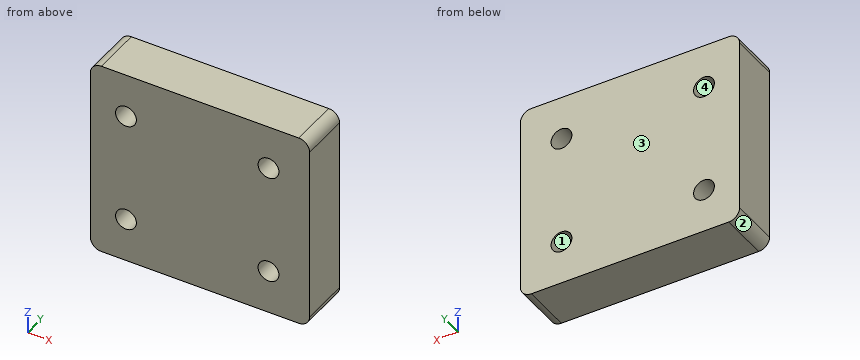
```python
from build123d import *

# Parameters (mm, degrees)
SKETCH1_W           = 40
SKETCH1_H           = 36
BOSS_EXTRUDE1_DEPTH = 9
SKETCH2_R           = 1.9
CUT_EXTRUDE1_DEPTH  = 10
FILLET1_R           = 2


with BuildPart() as part:
    # Sketch1 → Boss-Extrude1 (new body)
    with BuildSketch(Plane(origin=(0, 0, 0), x_dir=(1, 0, 0), z_dir=(0, 1, 0))):
        with Locations((9.482291419, -1.319229855)):
            Rectangle(SKETCH1_W, SKETCH1_H)
    extrude(amount=BOSS_EXTRUDE1_DEPTH)

    # Sketch2 → Cut-Extrude1 (cut)
    with BuildSketch(Plane(origin=(0, 9, 0), x_dir=(1, 0, 0), z_dir=(0, 1, 0))):
        with Locations(Location((-4.017708581, -11.319229855, 0), (0, 0, 270))):
            Circle(SKETCH2_R)
        with Locations(Location((21.982291419, -11.319229855, 0), (0, 0, 270))):
            Circle(SKETCH2_R)
        with Locations(Location((-4.017708581, 8.680770145, 0), (0, 0, 270))):
            Circle(SKETCH2_R)
        with Locations(Location((21.982291419, 8.680770145, 0), (0, 0, 270))):
            Circle(SKETCH2_R)
    extrude(amount=-CUT_EXTRUDE1_DEPTH, mode=Mode.SUBTRACT)

    # Fillet1
    fillet1_edges = [part.edges().sort_by_distance(p)[0] for p in [
        (-10.517708581, 4.5, -16.680770145),
        (29.482291419, 4.5, -16.680770145),
        (29.482291419, 4.5, 19.319229855),
        (-10.517708581, 4.5, 19.319229855),
    ]]
    fillet(fillet1_edges, radius=FILLET1_R)


solid = part.part
```
Geometry check sheet. Reference: the model listing, model coordinates, mm. Face numbers are marked on the shaded views. Round coordinates to 2 decimals unless told otherwise and drop trailing zeros. Loops run counter-clockwise (first coordinate to the right, second up) from the corner with the lowest first, then second, coordinate; pieces in that order, holes last. Notation, with made-up numbers: M -21,-1.5 L 4,-1.5 A11 cw 4,5.5 Z; hole C 43.5,48 d5. An arc over 180 degrees is marked long. Return JSON: item names as keys, results as strings. Group by question number.
(1) Section check A-A, the plane z = -7.5. Enter the section's corners in (x, y).
(2) Scan lines: line 1 along X through (y, z) = (6.75, -9.5); line 2 along Z through (x, y) = (21, 3.5); line 3 along X through (y, z) = (3.75, -8). Record each from-to range of solid material in increasing order. Write a range as [from, to].
(3) Section check B-B, the plane y = 4.5. Enter the section's corners in (x, z), and give its area (3 significant figures).
(4) Mould release check, pull along Z, two halves, no side actions. Record for the marked faces 1, 2, 3 and 4: pulls with the +Z half, pulls with the -Z half, needs draft (parallel to the pull), parting line crosses it, or undercut.
Data:
{
 "1": {"outline": "M -10.52,0 L -5.51,0 L -5.51,9 L -10.52,9 Z; M -2.53,0 L 20.49,0 L 20.49,9 L -2.53,9 Z; M 23.47,0 L 29.48,0 L 29.48,9 L 23.47,9 Z"},
 "2": {"line 1": "[-10.52, -5.73], [-2.3, 20.27], [23.7, 29.48]", "line 2": "[-16.68, -10.31], [-7.05, 9.69], [12.95, 19.32]", "line 3": "[-10.52, -5.79], [-2.24, 20.21], [23.76, 29.48]"},
 "3": {"outline": "M -10.52,-14.68 A2 ccw -8.52,-16.68 L 27.48,-16.68 A2 ccw 29.48,-14.68 L 29.48,17.32 A2 ccw 27.48,19.32 L -8.52,19.32 A2 ccw -10.52,17.32 Z; hole C -4.02,-8.68 d3.8; hole C -4.02,11.32 d3.8; hole C 21.98,-8.68 d3.8; hole C 21.98,11.32 d3.8", "area": "1,390 mm²"},
 "4": {"face 1": "undercut", "face 2": "pulls with the -Z half", "face 3": "needs draft", "face 4": "undercut"}
}
